from build123d import *

# Parameters (mm, degrees)
SKETCH1_R           = 51.054
SKETCH1_R_2         = 49.53
BOSS_EXTRUDE1_DEPTH = 381
SKETCH2_R           = 1.524
CUT_EXTRUDE1_DEPTH  = 136.398
CIRPATTERN1_COUNT   = 6
SKETCH3_R           = 1.524
CUT_EXTRUDE2_DEPTH  = 177.8
CIRPATTERN2_COUNT   = 6


with BuildPart() as part:
    # Sketch1 → Boss-Extrude1 (new body)
    with BuildSketch(Plane(origin=(0, 0, 0), x_dir=(1, 0, 0), z_dir=(0, 1, 0))):
        with Locations(Location((0, 0, 0), (0, 0, 270))):
            Circle(SKETCH1_R)
        with Locations(Location((0, 0, 0), (0, 0, 270))):
            Circle(SKETCH1_R_2, mode=Mode.SUBTRACT)
    extrude(amount=BOSS_EXTRUDE1_DEPTH)

    # Sketch2 → Cut-Extrude1 (cut)
    with BuildSketch(Plane(origin=(0, 0, 0), x_dir=(0, 0, -1), z_dir=(1, 0, 0))):
        with Locations((0, 19.05)):
            Circle(SKETCH2_R)
    cut_extrude1 = extrude(amount=-CUT_EXTRUDE1_DEPTH, mode=Mode.SUBTRACT)

    # CirPattern1: Cut-Extrude1 ×6 about axis
    cirpattern1_axis = Axis((0, 381, 0), (0, -1, 0))
    for i in range(1, CIRPATTERN1_COUNT):
        add(cut_extrude1.rotate(cirpattern1_axis, i * 360 / CIRPATTERN1_COUNT), mode=Mode.SUBTRACT)

    # Sketch3 → Cut-Extrude2 (cut)
    with BuildSketch(Plane(origin=(0, 0, 0), x_dir=(0, 0, -1), z_dir=(1, 0, 0))):
        with Locations((0, 368.3)):
            Circle(SKETCH3_R)
    cut_extrude2 = extrude(amount=-CUT_EXTRUDE2_DEPTH, mode=Mode.SUBTRACT)

    # CirPattern2: Cut-Extrude2 ×6 about axis
    cirpattern2_axis = Axis((0, 381, 0), (0, -1, 0))
    for i in range(1, CIRPATTERN2_COUNT):
        add(cut_extrude2.rotate(cirpattern2_axis, i * 360 / CIRPATTERN2_COUNT), mode=Mode.SUBTRACT)


solid = part.part
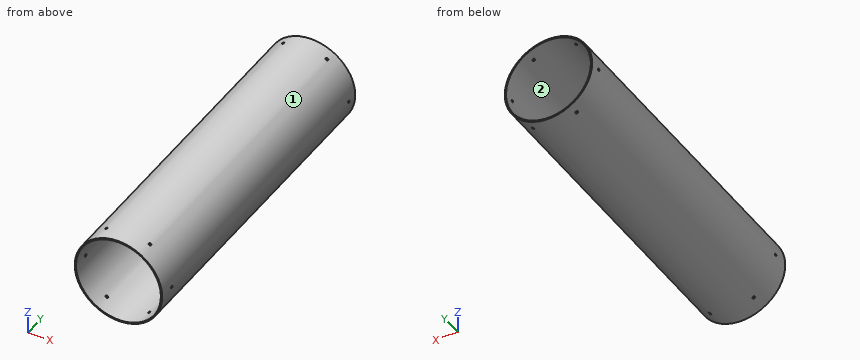
Check sheet for the modelled part. Datum: model origin and axes. Units: mm. Face numbers are marked on the shaded views. Give positions to 0.01 mm unless a question says otherwise; leave off trailing zeros. Write each loop counter-clockwise with the first axis right and the second up, starting at its lowest first coordinate (ties: lowest second). Pieces come first, ordered by that corner, then holes. Notation, with made-up numbers: M -30,44.5 L -4,44.5 A16 ccw -4,67.5 Z; hole C 31.25,-6 d2. An arc over 180 degrees is marked long. Use one line per item in the form item = value.
(1) Depth check by flat-ended pin: P1, Ø2, axis at x = -37, y = 296.5, coming from the +Z side; P2, Ø1, axis at y = 128, z = -6.5, coming from the -X side; P3, Ø8, axis at y = 265.5, z = -20.5, coming from the -X side. Enter the tip coordinate at first touch or a pass-through.
Answer block:
P1 = 36.2
P2 = -50.7
P3 = -48.31
(2) Section check A-A on x = 0. Record the boundary of the cut face in (y, z).
Answer block:
outline = M 0,-51.05 L 381,-51.05 L 381,-49.53 L 0,-49.53 Z; M 0,49.53 L 381,49.53 L 381,51.05 L 0,51.05 Z
(3) Material ranges on line 1 along Y through (x, z) = (-50.3, 0); line 2 along X through (y, z) = (109, 0); line 3 along X through (y, z) = (75, -2), recorded low to high.
Answer block:
line_1 = 0 to 17.53, 20.57 to 366.78, 369.82 to 381
line_2 = -51.05 to -49.53, 49.53 to 51.05
line_3 = -51.01 to -49.49, 49.49 to 51.01
(4) Section check B-B on z = 24. Record the boundary of the cut face in (x, y), plus the area to 3 significant figures.
Answer block:
outline = M -45.06,0 L -43.33,0 L -43.33,381 L -45.06,381 Z; M 43.33,0 L 45.06,0 L 45.06,381 L 43.33,381 Z
area = 1,320 mm2
(5) Section check C-C on y = 185. Record the boundary of the cut face in (x, z), plus the area to 3 significant figures.
Answer block:
outline = C 0,0 d102.11; hole C 0,0 d99.06
area = 482 mm2
(6) Draft check along X on the marked faces 1 and 2. Enter one of: pulls with the +X half, pulls with the -X half, needs draft (parallel to the pull), parting line crosses it, or undercut.
Answer block:
face_1 = parting line crosses it
face_2 = undercut
